Input: dimensioned drawing with shaded views. Units: mm. Origin: part minimum x, y, z. Give positions to 0.01 mm unless a question says otherwise; leave off trailing zeros. Write each loop counter-clockwise with the first axis right and the second up, starting at its lowest first coordinate (ties: lowest second). Pieces come first, ordered by that corner, then holes.
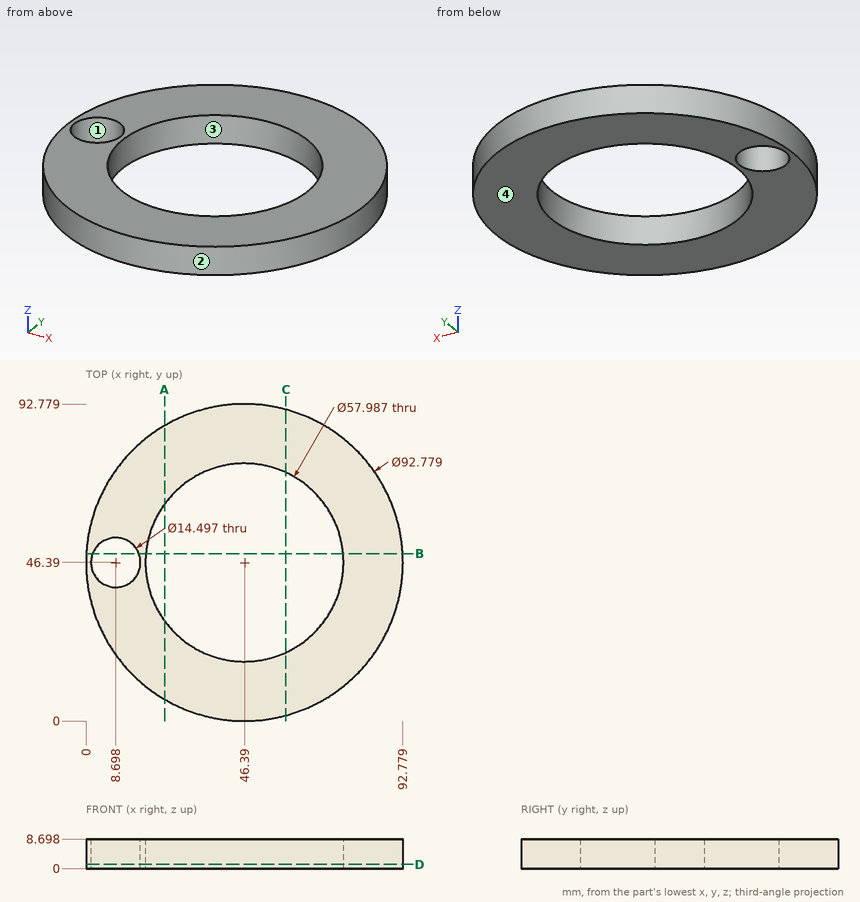
Item 1: Section A-A, the plane x = 23. Return the cut outline in (y, z), plus the area to 3 significant figures.
Found:
outline: (6.33, 0) - (29.26, 0) - (29.26, 8.7) - (6.33, 8.7) - close; (63.52, 0) - (86.45, 0) - (86.45, 8.7) - (63.52, 8.7) - close
area: 399 mm2
Item 2: Pull-direction query (Y, two-part tool) for the marked faces 1, 2, 3 and 4; classes: +Y half, -Y half, draft (parallel to the pull), parting line (faces both ways), or undercut.
Found:
face 1: undercut
face 2: parting line
face 3: undercut
face 4: draft
Item 3: Section D-D, the plane z = 1.25. Return the cut outline in (x, y).
Found:
outline: circle Ø92.78 at (46.39, 46.39); hole circle Ø14.5 at (8.7, 46.39); hole circle Ø57.99 at (46.39, 46.39)
Item 4: Section B-B, the plane y = 49. Return the cut outline in (x, z) (1 decimal).
Found:
outline: (0.1, 0) - (1.9, 0) - (1.9, 8.7) - (0.1, 8.7) - close; (15.5, 0) - (17.5, 0) - (17.5, 8.7) - (15.5, 8.7) - close; (75.3, 0) - (92.7, 0) - (92.7, 8.7) - (75.3, 8.7) - close
Item 5: Line query: L1, parallel to X at y = 35, z = 2.5; L2, parallel to X at y = 36, z = 1.25; L3, parallel to Y at x = 25.5, z = 3.25 (1 decimal). Output: solid intervals per line, ascending.
Found:
L1: x = 1.42 to 19.73, 73.05 to 91.36
L2: x = 1.18 to 19.32, 73.46 to 91.6
L3: y = 5 to 26.3, 66.5 to 87.8
Item 6: Pin query (flat end, axial travel): pin 1 Ø1.5 at (y, z) = (26, 3) entering from -X; pin 2 Ø1 at (y, z) = (27.5, 3.5) entering from -X; pin 3 Ø2 at (x, z) = (82, 2.5) entering from +Y. Return the tip coordinate at first contact, or that it passes through.
Found:
pin 1: stops at x = 4.36
pin 2: stops at x = 3.8
pin 3: stops at y = 77.28
Item 7: Section C-C, the plane x = 58.5. Return the cut outline in (y, z).
Found:
outline: (1.61, 0) - (20.05, 0) - (20.05, 8.7) - (1.61, 8.7) - close; (72.73, 0) - (91.17, 0) - (91.17, 8.7) - (72.73, 8.7) - close
